```python
from build123d import *

# Parameters (mm, degrees)
SKETCH1_W              = 34
SKETCH1_H              = 112
SKETCH1_R              = 1.5
BOARD_DEPTH            = 2
SKETCH2_W              = 16
SKETCH2_H              = 40
SKETCH2_W_2            = 6
SKETCH2_H_2            = 10
F_7SEG_DEPTH           = 11
SKETCH3_W              = 10
SKETCH3_H              = 20
SKETCH3_H_2            = 10
IC_DEPTH               = 8
SKETCH5_W              = 9
SKETCH5_H              = 17
BIENTROA_DEPTH         = 23
SKETCH6_R              = 3.4
BIENTROB_DEPTH         = 15
SKETCH7_W              = 10
SKETCH7_H              = 5
IRF540_DEPTH           = 26
SKETCH8_W              = 17
SKETCH8_H              = 10
DOMINO_DEPTH           = 10
SKETCH9_W              = 22
SKETCH9_H              = 30
EXTRUDE_7805_DEPTH     = 30
SPLIT2_SURFACE_1_BACK  = 127.76
SPLIT2_SURFACE_1_DEPTH = 255.52
SPLIT2_SURFACE_2_BACK  = 127.76
SPLIT2_SURFACE_2_DEPTH = 255.52


with BuildPart() as part:
    # Sketch1 → Board (new body)
    with BuildSketch(Plane(origin=(0, 0, 0), x_dir=(1, 0, 0), z_dir=(0, 1, 0))):
        Rectangle(SKETCH1_W, SKETCH1_H)
        with Locations(Location((13.6, -52.6, 0), (0, 0, 270))):
            Circle(SKETCH1_R, mode=Mode.SUBTRACT)
        with Locations(Location((-9, 49, 0), (0, 0, 270))):
            Circle(SKETCH1_R, mode=Mode.SUBTRACT)
        with Locations(Location((-9, 13, 0), (0, 0, 270))):
            Circle(SKETCH1_R, mode=Mode.SUBTRACT)
    extrude(amount=BOARD_DEPTH)

    # Sketch2 → 7SEG (add)
    with BuildSketch(Plane(origin=(0, 2, 0), x_dir=(1, 0, 0), z_dir=(0, 1, 0))):
        with Locations((4, 31)):
            Rectangle(SKETCH2_W, SKETCH2_H)
        with Locations((8, 5)):
            Rectangle(SKETCH2_W_2, SKETCH2_H_2)
    extrude(amount=F_7SEG_DEPTH)

    # Sketch3 → IC (add)
    with BuildSketch(Plane(origin=(0, 2, 0), x_dir=(1, 0, 0), z_dir=(0, 1, 0))):
        with Locations((-2, 26)):
            Rectangle(SKETCH3_W, SKETCH3_H)
        with Locations((4, 5)):
            Rectangle(SKETCH3_W, SKETCH3_H_2)
        with Locations((4, -17)):
            Rectangle(SKETCH3_W, SKETCH3_H_2)
    extrude(amount=IC_DEPTH)

    # Sketch5 → BienTroA (add)
    with BuildSketch(Plane(origin=(0, 2, 0), x_dir=(1, 0, 0), z_dir=(0, 1, 0))):
        with Locations((6.5, -14.5)):
            Rectangle(SKETCH5_W, SKETCH5_H)
    extrude(amount=BIENTROA_DEPTH)

    # Sketch6 → BienTroB (add)
    with BuildSketch(Plane(origin=(11, 0, 0), x_dir=(0, 0, -1), z_dir=(1, 0, 0))):
        with Locations(Location((-14.5, 16.6, 0), (0, 0, 180))):
            Circle(SKETCH6_R)
    extrude(amount=BIENTROB_DEPTH)

    # Sketch7 → IRF540 (add)
    with BuildSketch(Plane(origin=(0, 2, 0), x_dir=(1, 0, 0), z_dir=(0, 1, 0))):
        with Locations((5, -47.5)):
            Rectangle(SKETCH7_W, SKETCH7_H)
    extrude(amount=IRF540_DEPTH)

    # Sketch8 → Domino (add)
    with BuildSketch(Plane(origin=(0, 2, 0), x_dir=(1, 0, 0), z_dir=(0, 1, 0))):
        with Locations((-2.5, -50)):
            Rectangle(SKETCH8_W, SKETCH8_H)
    extrude(amount=DOMINO_DEPTH)

    # Sketch9 → 7805 (add)
    with BuildSketch(Plane(origin=(0, 2, 0), x_dir=(1, 0, 0), z_dir=(0, 1, 0))):
        with Locations((-13, -26)):
            Rectangle(SKETCH9_W, SKETCH9_H)
    extrude(amount=EXTRUDE_7805_DEPTH)


with BuildPart() as body_2:
    # Split2: the piece behind the surface
    add(part.part)
    # Split2 surface: a surface, the sketch's curves swept straight by 255.52 mm
    with BuildLine(Plane(origin=(0, 2, 0), x_dir=(1, 0, 0), z_dir=(0, 1, 0)).offset(-SPLIT2_SURFACE_1_BACK), mode=Mode.PRIVATE) as split2_surface_1_path:
        Line((17, 11), (-17, 11))
    split2_surface_1 = Shell.extrude(split2_surface_1_path.wire(), (0 * SPLIT2_SURFACE_1_DEPTH, 1 * SPLIT2_SURFACE_1_DEPTH, 0 * SPLIT2_SURFACE_1_DEPTH))
    split(bisect_by=split2_surface_1, keep=Keep.BOTTOM)


with BuildPart() as part_1:
    add(part.part)

    # Split2: split by a surface, the side it looks to stays
    # Split2 surface: a surface, the sketch's curves swept straight by 255.52 mm
    with BuildLine(Plane(origin=(0, 2, 0), x_dir=(1, 0, 0), z_dir=(0, 1, 0)).offset(-SPLIT2_SURFACE_2_BACK), mode=Mode.PRIVATE) as split2_surface_2_path:
        Line((17, 11), (-17, 11))
    split2_surface_2 = Shell.extrude(split2_surface_2_path.wire(), (0 * SPLIT2_SURFACE_2_DEPTH, 1 * SPLIT2_SURFACE_2_DEPTH, 0 * SPLIT2_SURFACE_2_DEPTH))
    split(bisect_by=split2_surface_2, keep=Keep.TOP)


solid = body_2.part
```
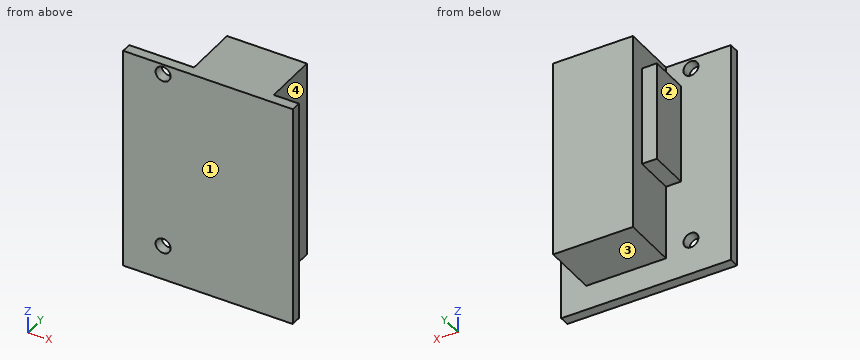
Model file for the job. Use its own axes, mm. Face numbers are marked on the shaded views. A direction names the side the tool comes from. Give positions to 0.01 mm unless a question says otherwise; leave off trailing zeros. Loops run counter-clockwise (first coordinate to the right, second up) from the corner with the lowest first, then second, coordinate; pieces in that order, holes last. Notation, with made-up numbers: (40, 51) - (58, 51) arc R28 cw to (58, 76) - close; hole circle Ø3 at (64.25, 45). An arc over 180 degrees is marked (long way). One line per item, written item: value. Start each with the question number.
1. Slice it at D-D (x = 0.5). List the corners of the cut face in (y, z), plus the area to 3 significant figures.
2. Which spindle directions (+Z, -Z, +X, -X, +Y, -Y) get a long thin tool onto all of the face, cutting with end or side? Do the marked faces 1, 2, 3 and 4. Say none if no direction does.
3. Slice it at B-B (y = 5.75). List the corners of the cut face in (x, z), plus the area to 3 significant figures.
4. Slice it at C-C (z = -37). List the corners of the cut face in (x, y), plus the area to 3 significant figures.
5. Probe L1, parallel to X at y = 0.5, z = -49; L2, parallel to X at y = 10.5, z = -22.5; L3, parallel to Y at x = -13, z = -39. List the from-to ranges inside material, lowest first. Write a range as from..to.
6. Slice it at A-A (z = -49). List the corners of the cut face in (x, y), plus the area to 3 significant figures.
7. Pin check, flat tips, straight feed: pin 1 (4 mm diameter, centred on y = 8, z = -28, fed in from +X); pin 2 (3.5 mm diameter, centred on x = -9, z = -13, fed in from +Y); pin 3 (5.5 mm diameter, centred on x = 2.5, y = 7, fed in from -Z). Stop position of each tip, or through.
Solution:
1. outline: (0, -56) - (2, -56) - (2, -51) - (13, -51) - (13, -11) - (0, -11) - close
1. area: 530 mm^2
2. face 1: +Z, -Z, +X, -X, -Y
2. face 2: +Z, -Z, -X, +Y
2. face 3: -Z, +X, -X, +Y
2. face 4: +Z, -Z, +X, +Y
3. outline: (-7, -36) - (-4, -36) - (-4, -51) - (12, -51) - (12, -11) - (-4, -11) - (-4, -16) - (-7, -16) - close
3. area: 700 mm^2
4. outline: (-17, 0) - (17, 0) - (17, 2) - (12, 2) - (12, 13) - (-4, 13) - (-4, 2) - (-17, 2) - close
4. area: 244 mm^2
5. L1: x = -17..-10.5, -7.5..17
5. L2: x = -4..12
5. L3: y = 0..2
6. outline: (-17, 0) - (-10.5, 0) - (-10.5, 2) - (-17, 2) - close; (-7.5, 0) - (17, 0) - (17, 2) - (12, 2) - (12, 13) - (-4, 13) - (-4, 2) - (-7.5, 2) - close
6. area: 238 mm^2
7. pin 1: stops at x = 12
7. pin 2: stops at y = 2
7. pin 3: stops at z = -51
